from build123d import *

# Parameters (mm, degrees)
SKETCH1_R               = 2.5
BOSS_EXTRUDE1_DEPTH     = 4
SKETCH2_R               = 5
BOSS_EXTRUDE2_DEPTH     = 0.75
M1_6_NUT_DEPTH          = 9.124038405
M1_6_NUT_DEPTH_BACK     = 9.124038405
CUT_EXTRUDE1_DEPTH      = 10.883671537
CUT_EXTRUDE1_DEPTH_BACK = 10.883671537
SKETCH5_W               = 6.5
SKETCH5_H               = 0.25


with BuildPart() as part:
    # Sketch1 → Boss-Extrude1 (new, symmetric)
    with BuildSketch(Plane(origin=(0, 0, 0), x_dir=(0, 0, -1), z_dir=(1, 0, 0))):
        Circle(SKETCH1_R)
    extrude(amount=BOSS_EXTRUDE1_DEPTH, both=True)

    # Sketch2 → Boss-Extrude2 (add)
    with BuildSketch(Plane(origin=(4, 0, 0), x_dir=(0, 0, -1), z_dir=(1, 0, 0))):
        Circle(SKETCH2_R)
    boss_extrude2 = extrude(amount=-BOSS_EXTRUDE2_DEPTH)

    # Mirror1: Boss-Extrude2 across plane
    add(boss_extrude2.mirror(Plane(origin=(0, 0, 0), x_dir=(0, 0, 1), z_dir=(1, 0, 0))))

    # Sketch3 → M1.6 Nut (cut, two sides: drawn at the far end of the back side and taken through both)
    with BuildSketch(Plane(origin=(0, 0, 0), x_dir=(0, 0, -1), z_dir=(1, 0, 0)).offset(-M1_6_NUT_DEPTH_BACK)):
        Polygon((1.75, 0), (1.75, 1.010362971), (0.875, 1.515544457), (0, 2.020725942), (-0.875, 1.515544457), (-1.75, 1.010362971), (-1.75, 0), (-1.75, -1.010362971), (-0.875, -1.515544457), (0, -2.020725942), (0.875, -1.515544457), (1.75, -1.010362971), align=None)
    extrude(amount=M1_6_NUT_DEPTH + M1_6_NUT_DEPTH_BACK, mode=Mode.SUBTRACT)

    # Sketch5 → Cut-Extrude1 (cut, two sides: drawn at the far end of the back side and taken through both)
    with BuildSketch(Plane(origin=(0, 1.010362971, -1.75), x_dir=(1, 0, 0), z_dir=(0, -0.8660254037844384, 0.5000000000000007)).offset(-CUT_EXTRUDE1_DEPTH_BACK)):
        with Locations((0, 2.520725942)):
            Rectangle(SKETCH5_W, SKETCH5_H)
    extrude(amount=CUT_EXTRUDE1_DEPTH + CUT_EXTRUDE1_DEPTH_BACK, mode=Mode.SUBTRACT)


solid = part.part
Input: part model. Units: mm. Frame: model coordinates. A direction names the side the tool comes from. Give positions to 0.01 mm unless a question says otherwise; leave off trailing zeros. Loops run counter-clockwise (first coordinate to the right, second up) from the corner with the lowest first, then second, coordinate; pieces in that order, holes last. Notation, with made-up numbers: (88.25, 1) -> (133.25, 1) arc R14 cw to (133.25, 23) -> close; hole circle Ø2 at (3.25, 16.5). An arc over 180 degrees is marked (long way). Answer as a JSON object with one key per item and string values. Group by question number.
Item 1: Line query: probe 1 along X at (y, z) = (-2.75, 2.5); probe 2 along Y at (x, z) = (-1, -0.5); probe 3 along Y at (x, z) = (1.25, 1). Output: solid intervals per line, ascending.
Item 2: Cut plane A-A, the plane x = 2.75. Return the cut outline in (y, z) (3 decimals), and give its area (3 significant figures).
Item 3: Pin query (flat end, axial travel): P1, Ø2, axis at x = -0.5, z = 2.5, coming from the -Y side; P2, Ø1, axis at x = 1, y = 0.5, coming from the -Z side; P3, Ø4, axis at x = -1, z = -2, coming from the -Y side. Return the tip coordinate at first contact, or that it passes through.
Item 4: Pull-direction query (X, two-part tool) for faces 1 (the cylindrical face through (0.05, -1.31, -2.13)), 2 (the flat face through (-4, -2.2, 0.1)), 3 (the cylindrical face through (0.046, 1.276, 2.15)), 4 (the flat face through (0, 0, -1.75)); classes: released by +X, released by -X, zero draft, split by the parting line, or undercut.
Item 5: Cut plane D-D, the plane y = 0. Return the cut outline in (x, z).
Item 6: Reachability of faces 5 (the flat face through (-0.1, 0.5, 1.75)), 6 (the flat face through (4, -2.2, 0.1)), 7 (the flat face through (-0.05, 2.08, 0.4)) from +Z, -Z, +X, -X, +Y, -Y: full face, straight path, thin tool, end or side. Return the list, or none.
Item 7: Cut plane B-B, the plane y = 3. Return the cut outline in (x, z).
Item 8: Cut plane C-C, the plane z = 3.75. Return the cut outline in (x, y).
Checks:
{
 "1": {"probe 1": "x = -4 to -3.25, 3.25 to 4", "probe 2": "y = -2.45 to -1.73, 1.73 to 2.45", "probe 3": "y = -2.29 to -1.44, 1.54 to 2.29"},
 "2": {"outline": "(-2.021, 0) -> (-1.01, 1.75) -> (-0.26, 1.75) -> (-1.11, 2.24) arc R2.5 ccw (long way) to (2.495, 0.159) -> (1.646, 0.65) -> (2.021, 0) -> (1.01, -1.75) -> (-1.01, -1.75) -> close; (-0.82, 2.362) -> (0.24, 1.75) -> (1.01, 1.75) -> (1.396, 1.083) -> (2.455, 0.471) arc R2.5 ccw to start", "area": "8.47 mm²"},
 "3": {"P1": "stops at y = -2", "P2": "stops at z = -2.5", "P3": "stops at y = -2.5"},
 "4": {"face 1": "undercut", "face 2": "released by -X", "face 3": "undercut", "face 4": "zero draft"},
 "5": {"outline": "(-4, -5) -> (-3.25, -5) -> (-3.25, -2.5) -> (3.25, -2.5) -> (3.25, -5) -> (4, -5) -> (4, -1.75) -> (-4, -1.75) -> close; (-4, 1.75) -> (-3.25, 1.75) -> (-3.25, 1.89) -> (3.25, 1.89) -> (3.25, 1.75) -> (4, 1.75) -> (4, 5) -> (3.25, 5) -> (3.25, 2.5) -> (-3.25, 2.5) -> (-3.25, 5) -> (-4, 5) -> close"},
 "6": {"face 5": "+X, -X", "face 6": "+Z, -Z, +X, +Y, -Y", "face 7": "none"},
 "7": {"outline": "(-4, -4) -> (-3.25, -4) -> (-3.25, 4) -> (-4, 4) -> close; (3.25, -4) -> (4, -4) -> (4, 4) -> (3.25, 4) -> close"},
 "8": {"outline": "(-4, -3.31) -> (-3.25, -3.31) -> (-3.25, 3.31) -> (-4, 3.31) -> close; (3.25, -3.31) -> (4, -3.31) -> (4, 3.31) -> (3.25, 3.31) -> close"}
}
